Autodesk Inventor part; units mm, degrees
ref_plane "YZ Plane" through (0, 0, 0) normal (1, 0, 0) x (0, 1, 0)
ref_plane "XZ Plane" through (0, 0, 0) normal (0, 1, 0) x (-1, 0, 0)
ref_plane "XY Plane" through (0, 0, 0) normal (0, 0, 1) x (1, 0, 0)
sketch "Sketch1" plane through (60.3372, -82.808, 0) normal (0, 0, 1) x (1, 0, 0)
  circle A0 centre (0, 0) radius 20.32 construction
  circle A1 centre (0, 0) radius 22.86 construction
  circle A2 centre (24.5471, 44.4756) radius 30.48 construction
  circle A3 centre (-36.4129, 44.4756) radius 30.48 construction
  circle A4 centre (-36.4129, 44.4756) radius 33.02 construction
  line L0 (-15.4952, 18.9262) -> (-14.4815, 17.688)
  circle A5 centre (24.5471, 44.4756) radius 33.02 construction
  circle A6 centre (24.5471, 44.4756) radius 14.2875
  circle A7 centre (-36.4129, 44.4756) radius 14.2875
  circle A8 centre (0, 0) radius 14.2875
  circle A9 centre (24.5471, 44.4756) radius 19.1008 construction
  circle A10 centre (24.5471, 44.4756) radius 21.0058 construction
  circle A11 centre (-36.4129, 44.4756) radius 19.1008 construction
  circle A12 centre (-36.4129, 44.4756) radius 21.0058 construction
  line L1 (-36.4129, 44.4756) -> (-174.0993, 152.048) construction
  line L2 (24.5471, 44.4756) -> (162.2336, 152.048) construction
  circle A13 centre (-174.0993, 152.048) radius 14.2875
  circle A14 centre (162.2336, 152.048) radius 14.2875
  circle A15 centre (-174.0993, 152.048) radius 22.225 construction
  circle A16 centre (162.2336, 152.048) radius 22.225 construction
  line L3 (-160.4162, 169.5616) -> (-45.921, 80.1081)
  line L4 (-42.9811, 79.0958) -> (31.1154, 79.0958)
  arc A17 (31.1154, 79.0958) -> (34.0553, 80.1081) centre (31.1154, 83.871) ccw
  arc A18 (-45.921, 80.1081) -> (-42.9811, 79.0958) centre (-42.9811, 83.871) ccw
  line L5 (34.0553, 80.1081) -> (148.5505, 169.5616)
  line L6 (-36.4129, 79.0958) -> (-36.4129, 77.4956) construction
  arc A19 (177.8656, 136.2496) -> (148.5505, 169.5616) centre (162.2336, 152.048) ccw
  arc A20 (-160.4162, 169.5616) -> (-189.2001, 135.7411) centre (-174.0993, 152.048) ccw
  circle A21 centre (-105.2561, 98.2618) radius 2.4892
  circle A22 centre (0, -30.8102) radius 6.35 construction
  circle A23 centre (0, -30.8102) radius 2.4892
  line L7 (0, -22.86) -> (0, -24.4602)
  line L8 (-189.2001, 135.7411) -> (-4.3145, -35.4693)
  line L9 (177.8656, 136.2496) -> (4.4663, -35.324)
  arc A24 (-4.3145, -35.4693) -> (4.4663, -35.324) centre (0, -30.8102) ccw
  circle A25 centre (-105.2561, 98.2618) radius 6.35 construction
  circle A26 centre (93.3904, 98.2618) radius 6.35 construction
  circle A27 centre (93.3904, 98.2618) radius 2.4892
  circle A28 centre (-174.0993, 152.048) radius 50.8 construction
  circle A29 centre (162.2336, 152.048) radius 50.8 construction
  line L10 (-333.708, 192.5945) -> (-312.3217, 152.048) construction
  dimension "d25" = 40.64
  dimension "d24" = 2.54
  dimension "d23" = 60.96
  dimension "d22" = 2.54
  dimension "d21" = 1.6002
  dimension "d20" = 28.575
  dimension "d19" = 38.2016
  dimension "d18" = 42.0116
  dimension "d17" = 174.7266
  dimension "d16" = 104
  dimension "d15" = 28.575
  dimension "d14" = 44.45
  dimension "d13" = 44.45
  dimension "d12" = 4.7752
  dimension "d11" = 1.6002
  dimension "d9" = 4.9784
  dimension "d8" = 12.7
  dimension "d7" = 4.9784
  dimension "d6" = 1.6002
  dimension "d5" = 12.7
  dimension "d3" = 12.7
  dimension "d2" = 4.9784
  dimension "d10" = 87.3633
  dimension "d4" = 87.3633
  dimension "d0" = 101.6
  dimension "d1" = 101.6
extrude "Extrusion1" add sketch "Sketch1" along normal mid plane 6.35
properties part number "Gearbox #2 Top Plate"
Model file for the job. Use its own axes, mm. A direction names the side the tool comes from. Give positions to 0.01 mm unless a question says otherwise; leave off trailing zeros. Order: outer loops, then holes, each group sorted by start corner. A loop starts at its lowest first (then second) coordinate and runs counter-clockwise, first axis right, second up. Notation, with made-up numbers: M -3,-29.75 L 47,-29.75 A35 ccw 47,4.25 Z; hole C -39,-14 d6. An arc over 180 degrees is marked long. Put each result on its own line as item: value. Start each with the question number.
(1) Drill centre lines: L1, parallel to X at y = -37, z = -1.5; L2, parallel to X at y = 73, z = 2.25; L3, parallel to X at y = 77.5, z = 1.75. Where is each one in solid material? Low to high. Write a range as [from, to].
(2) Tool access for faces 5 (the face through (-100.564, 74.712, -0.044)), 6 (the face through (-43.63, 42.65, -0.04)): list every direction of +Z, -Z, +X, -X, +Y, -Y with a clear straight run to the whole face (end or side of a thin tool).
(3) Band-saw the part on B-B on y = -31. Give the cut face in (x, z) (3 decimals), then the cut area to 3 significant figures.
(4) Band-saw the part on A-A on y = 69.24. Give the cut face in (x, z) (3 decimals).
(5) Band-saw the part on D-D on x = 5.5. Give the cut face in (y, z) (3 decimals).
(6) Band-saw the part on C-C on z = -0.75. Count the separate pieces of the cut face and the enclosed holes in it, then the cut area to 3 significant figures.
(7) Pull direction X, two halves, no side cores. Call faces 1 (the face through (58.477, -96.974, -0.044)), 2 (the face through (54, -6, 3.175)), 3 (the face through (-37.714, -31.474, -0.044)), 4 (the face through (152.72, -31.14, -0.04)): released by +X, released by -X, zero draft, split by the parting line, or undercut.
(8) Pin check, flat tips, straight feed: pin 1 Ø3 at (y, z) = (-81.5, 1.5) entering from +X; pin 2 Ø1 at (x, z) = (41.5, -1.5) entering from -Y; pin 3 Ø23 at (x, y) = (60.34, -82.81) entering from -Z; pin 4 Ø8 at (x, y) = (153.73, 15.45) entering from +Z (3 decimals). Stop position of each tip, or through.
Results below:
1. L1: x = [-31.75, 9.7], [38.15, 70.66], [99.11, 146.8]
1. L2: x = [-135.67, -127.55], [-99.98, -82.48], [191.28, 208.79], [236.35, 244.48]
1. L3: x = [-134.4, -125.42], [-102.1, -88.23], [197.04, 210.91], [234.23, 243.2]
2. face 5: +Z, -Z
2. face 6: +Z, -Z, +Y
3. outline: M -38.226,-3.175 L 11.662,-3.175 L 11.662,3.175 L -38.226,3.175 Z; M 36.187,-3.175 L 72.622,-3.175 L 72.622,3.175 L 36.187,3.175 Z; M 97.147,-3.175 L 152.863,-3.175 L 152.863,3.175 L 97.147,3.175 Z
3. area: 902 mm2
4. outline: M -135.987,-3.175 L -128.05,-3.175 L -128.05,3.175 L -135.987,3.175 Z; M -99.475,-3.175 L -77.663,-3.175 L -77.663,3.175 L -99.475,3.175 Z; M 186.471,-3.175 L 208.283,-3.175 L 208.283,3.175 L 186.471,3.175 Z; M 236.858,-3.175 L 244.796,-3.175 L 244.796,3.175 L 236.858,3.175 Z
5. outline: M -71.492,-3.175 L 4.266,-3.175 L 4.266,3.175 L -71.492,3.175 Z
6. separate pieces: 1
6. enclosed holes: 8
6. area: 24,300 mm2
7. face 1: undercut
7. face 2: zero draft
7. face 3: released by -X
7. face 4: released by +X
8. pin 1: stops at x = 103.34
8. pin 2: stops at y = -105.29
8. pin 3: passes through
8. pin 4: stops at z = 3.175
